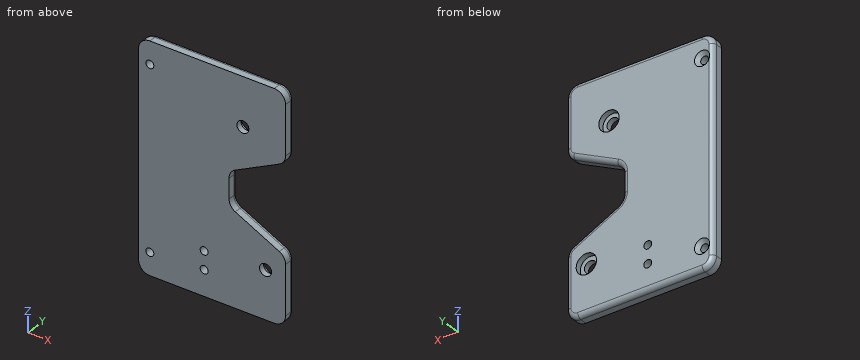
from build123d import *

# Parameters (mm, degrees)
SKETCH2_W           = 65
SKETCH2_H           = 100
SKETCH2_R           = 1.75
SKETCH2_R_2         = 2.65
BOSS_EXTRUDE1_DEPTH = 5
SKETCH3_R           = 4.5
CUT_EXTRUDE1_DEPTH  = 2.5
CUT_EXTRUDE2_DEPTH  = 60.843546018
FILLET1_R           = 5
CHAMFER1_SIZE       = 1.6
FILLET3_R           = 5
FILLET2_R           = 2
SKETCH5_R           = 1.75
CUT_EXTRUDE3_DEPTH  = 60.843546072


with BuildPart() as part:
    # Sketch2 → Boss-Extrude1 (new body)
    with BuildSketch(Plane(origin=(0, 0, 0), x_dir=(1, 0, 0), z_dir=(0, 1, 0))):
        Rectangle(SKETCH2_W, SKETCH2_H)
        with Locations(Location((-27.5, 40, 0), (0, 0, 270))):
            Circle(SKETCH2_R, mode=Mode.SUBTRACT)
        with Locations(Location((-27.5, -40, 0), (0, 0, 270))):
            Circle(SKETCH2_R, mode=Mode.SUBTRACT)
        with Locations(Location((23.6525, 28.725, 0), (0, 0, 270))):
            Circle(SKETCH2_R_2, mode=Mode.SUBTRACT)
        with Locations(Location((13.65, -28.4925, 0), (0, 0, 270))):
            Circle(SKETCH2_R_2, mode=Mode.SUBTRACT)
    extrude(amount=BOSS_EXTRUDE1_DEPTH)

    # Sketch3 → Cut-Extrude1 (cut)
    with BuildSketch(Plane(origin=(0, 5, 0), x_dir=(1, 0, 0), z_dir=(0, 1, 0))):
        with Locations(Location((23.6525, 28.725, 0), (0, 0, 270))):
            Circle(SKETCH3_R)
        with Locations(Location((13.65, -28.4925, 0), (0, 0, 270))):
            Circle(SKETCH3_R)
    extrude(amount=-CUT_EXTRUDE1_DEPTH, mode=Mode.SUBTRACT)

    # Sketch4 → Cut-Extrude2 (cut, through all)
    with BuildSketch(Plane(origin=(0, 5, 0), x_dir=(1, 0, 0), z_dir=(0, 1, 0))):
        Polygon((7.5, 7.5), (7.5, -7.5), (32.5, -20), (32.5, 20), align=None)
    extrude(amount=-CUT_EXTRUDE2_DEPTH, mode=Mode.SUBTRACT)

    # Fillet1
    fillet1_edges = [part.edges().sort_by_distance(p)[0] for p in [
        (32.5, 2.5, 50),
        (-32.5, 2.5, 50),
        (-32.5, 2.5, -50),
        (32.5, 2.5, -50),
    ]]
    fillet(fillet1_edges, radius=FILLET1_R)

    # Chamfer1
    chamfer1_edges = [part.edges().sort_by_distance(p)[0] for p in [
        (-27.5, 5, -41.75),
        (-27.5, 5, 38.25),
    ]]
    chamfer(chamfer1_edges, length=CHAMFER1_SIZE)

    # Fillet3
    fillet3_edges = [part.edges().sort_by_distance(p)[0] for p in [
        (7.5, 2.5, -7.5),
        (32.5, 2.5, -20),
        (32.5, 2.5, 20),
        (7.5, 2.5, 7.5),
    ]]
    fillet(fillet3_edges, radius=FILLET3_R)

    # Fillet2
    # the kernel refuses this fillet: 2 mm, written as the material it takes off along each edge
    with BuildSketch(Plane(origin=(12.5, 5, 4.409830056), x_dir=(-0.447213595499958, 0, 0.894427190999916), z_dir=(0.894427190999916, 0, 0.447213595499958))) as fillet2_piece_1:
        with BuildLine():
            CenterArc((5 + FILLET2_R, FILLET2_R), FILLET2_R, 180, 90)
            Line((5, FILLET2_R), (5, 0))
            Line((5, 0), (5 + FILLET2_R, 0))
        make_face()
    revolve(axis=Axis((12.5, 5, 4.409830056), (0, -1, 0)), revolution_arc=63.434948823, mode=Mode.SUBTRACT)
    with BuildSketch(Plane(origin=(12.5, 5, -4.409830056), x_dir=(-0.447213595499958, 0, -0.894427190999916), z_dir=(0.894427190999916, 0, -0.447213595499958))) as fillet2_piece_2:
        with BuildLine():
            CenterArc((5 + FILLET2_R, -FILLET2_R), FILLET2_R, 90, 90)
            Line((5, -FILLET2_R), (5, 0))
            Line((5, 0), (5 + FILLET2_R, 0))
        make_face()
    revolve(axis=Axis((12.5, 5, -4.409830056), (0, 1, 0)), revolution_arc=63.434948823, mode=Mode.SUBTRACT)
    with BuildSketch(Plane(origin=(32.5, 5, 23.090169944), x_dir=(-1, 0, 0), z_dir=(0, 0, 1)), Plane(origin=(32.5, 5, -45), x_dir=(-1, 0, 0), z_dir=(0, 0, 1))) as fillet2_piece_3:
        with BuildLine():
            CenterArc((FILLET2_R, FILLET2_R), FILLET2_R, 180, 90)
            Line((0, FILLET2_R), (0, 0))
            Line((0, 0), (FILLET2_R, 0))
        make_face()
    extrude(amount=21.909830056, mode=Mode.SUBTRACT)
    with BuildSketch(Plane(origin=(27.5, 5, 50), x_dir=(0, 0, -1), z_dir=(-1, 0, 0)), Plane(origin=(-27.5, 5, -50), x_dir=(0, 0, 1), z_dir=(1, 0, 0))) as fillet2_piece_4:
        with BuildLine():
            CenterArc((FILLET2_R, FILLET2_R), FILLET2_R, 180, 90)
            Line((0, FILLET2_R), (0, 0))
            Line((0, 0), (FILLET2_R, 0))
        make_face()
    extrude(amount=55, mode=Mode.SUBTRACT)
    with BuildSketch(Plane(origin=(-32.5, 5, 45), x_dir=(1, 0, 0), z_dir=(0, 0, -1))) as fillet2_piece_5:
        with BuildLine():
            CenterArc((FILLET2_R, FILLET2_R), FILLET2_R, 180, 90)
            Line((0, FILLET2_R), (0, 0))
            Line((0, 0), (FILLET2_R, 0))
        make_face()
    extrude(amount=90, mode=Mode.SUBTRACT)
    with BuildSketch(Plane(origin=(-27.5, 5, 45), x_dir=(-1, 0, 0), z_dir=(0, 0, -1))) as fillet2_piece_6:
        with BuildLine():
            CenterArc((5 - FILLET2_R, -FILLET2_R), FILLET2_R, 0, 90)
            Line((5, -FILLET2_R), (5, 0))
            Line((5, 0), (5 - FILLET2_R, 0))
        make_face()
    revolve(axis=Axis((-27.5, 5, 45), (0, 1, 0)), revolution_arc=90, mode=Mode.SUBTRACT)
    with BuildSketch(Plane(origin=(27.5, 5, -45), x_dir=(0, 0, -1), z_dir=(-1, 0, 0))) as fillet2_piece_7:
        with BuildLine():
            CenterArc((5 - FILLET2_R, FILLET2_R), FILLET2_R, 270, 90)
            Line((5, FILLET2_R), (5, 0))
            Line((5, 0), (5 - FILLET2_R, 0))
        make_face()
    revolve(axis=Axis((27.5, 5, -45), (0, -1, 0)), revolution_arc=90, mode=Mode.SUBTRACT)
    with BuildSketch(Plane(origin=(-27.5, 5, -45), x_dir=(0, 0, -1), z_dir=(1, 0, 0))) as fillet2_piece_8:
        with BuildLine():
            CenterArc((5 - FILLET2_R, -FILLET2_R), FILLET2_R, 0, 90)
            Line((5, -FILLET2_R), (5, 0))
            Line((5, 0), (5 - FILLET2_R, 0))
        make_face()
    revolve(axis=Axis((-27.5, 5, -45), (0, 1, 0)), revolution_arc=90, mode=Mode.SUBTRACT)
    with BuildSketch(Plane(origin=(27.5, 5, 45), x_dir=(0, 0, 1), z_dir=(-1, 0, 0))) as fillet2_piece_9:
        with BuildLine():
            CenterArc((5 - FILLET2_R, -FILLET2_R), FILLET2_R, 0, 90)
            Line((5, -FILLET2_R), (5, 0))
            Line((5, 0), (5 - FILLET2_R, 0))
        make_face()
    revolve(axis=Axis((27.5, 5, 45), (0, 1, 0)), revolution_arc=90, mode=Mode.SUBTRACT)
    with BuildSketch(Plane(origin=(29.736067977, 5, -18.618033989), x_dir=(-0.4472135954999579, 0, -0.8944271909999159), z_dir=(-0.894427190999916, 0, 0.4472135954999579)), Plane(origin=(10.263932023, 5, 8.881966011), x_dir=(-0.4472135954999579, 0, 0.894427190999916), z_dir=(0.894427190999916, 0, 0.4472135954999579))) as fillet2_piece_10:
        with BuildLine():
            CenterArc((FILLET2_R, FILLET2_R), FILLET2_R, 180, 90)
            Line((0, FILLET2_R), (0, 0))
            Line((0, 0), (FILLET2_R, 0))
        make_face()
    extrude(amount=21.770509831, mode=Mode.SUBTRACT)
    with BuildSketch(Plane(origin=(7.5, 5, -4.409830056), x_dir=(-1, 0, 0), z_dir=(0, 0, 1))) as fillet2_piece_11:
        with BuildLine():
            CenterArc((FILLET2_R, FILLET2_R), FILLET2_R, 180, 90)
            Line((0, FILLET2_R), (0, 0))
            Line((0, 0), (FILLET2_R, 0))
        make_face()
    extrude(amount=8.819660113, mode=Mode.SUBTRACT)
    with BuildSketch(Plane(origin=(27.5, 5, 23.090169944), x_dir=(1, 0, 0), z_dir=(0, 0, 1))) as fillet2_piece_12:
        with BuildLine():
            CenterArc((5 - FILLET2_R, -FILLET2_R), FILLET2_R, 0, 90)
            Line((5, -FILLET2_R), (5, 0))
            Line((5, 0), (5 - FILLET2_R, 0))
        make_face()
    revolve(axis=Axis((27.5, 5, 23.090169944), (0, 1, 0)), revolution_arc=63.434948823, mode=Mode.SUBTRACT)
    with BuildSketch(Plane(origin=(27.5, 5, -23.090169944), x_dir=(1, 0, 0), z_dir=(0, 0, -1))) as fillet2_piece_13:
        with BuildLine():
            CenterArc((5 - FILLET2_R, FILLET2_R), FILLET2_R, 270, 90)
            Line((5, FILLET2_R), (5, 0))
            Line((5, 0), (5 - FILLET2_R, 0))
        make_face()
    revolve(axis=Axis((27.5, 5, -23.090169944), (0, -1, 0)), revolution_arc=63.434948823, mode=Mode.SUBTRACT)

    # Sketch5 → Cut-Extrude3 (cut, through all)
    with BuildSketch(Plane(origin=(0, 5, 0), x_dir=(1, 0, 0), z_dir=(0, 1, 0))):
        with Locations(Location((-3.507863002, 38.632025627, 0), (0, 0, 270))):
            Circle(SKETCH5_R)
        with Locations(Location((-3.507863002, 30.632025627, 0), (0, 0, 270))):
            Circle(SKETCH5_R)
    extrude(amount=-CUT_EXTRUDE3_DEPTH, mode=Mode.SUBTRACT)


solid = part.part
Verification items for the finished model (mm, model axes). Coordinates: 2 decimals unless noted, no trailing zeros. One line per item, written item: value. Start each with the question number.
Item 1: Sectioned sample at A-A (x = 12.5). Count the separate pieces of the cut face and the enclosed holes in it, then the cut area to 3 significant figures.
Item 2: Scan lines: probe 1 along X at (y, z) = (2.45, -31); probe 2 along Z at (x, y) = (13.65, 0.5) (1 decimal); probe 3 along X at (y, z) = (2.65, -40). Record each from-to range of solid material in increasing order.
Item 3: Gauge pin test, flat ends, axial feed: pin 1 (5.5 mm diameter, centred on x = -27.5, z = -40, fed in from +Y); pin 2 (2 mm diameter, centred on x = -3.51, z = -38.63, fed in from -Y); pin 3 (6 mm diameter, centred on x = 13.65, z = 28.49, fed in from +Y). Record the tip position at first contact, or that the pin passes through.
Conclusion:
1. separate pieces: 3
1. enclosed holes: 0
1. area: 363 mm^2
2. probe 1: x = -32.5 to -5.22, -1.8 to 22.29, 25.01 to 32.5
2. probe 2: z = -50 to -10.6, 10.6 to 25.8, 31.1 to 50
2. probe 3: x = -32.5 to -29.25, -25.75 to -4.6, -2.42 to 32.5
3. pin 1: stops at y = 4.4
3. pin 2: passes through
3. pin 3: stops at y = 2.5
